```python
from build123d import *

# Parameters (mm, degrees)
SKETCH1_R           = 6
BOSS_EXTRUDE1_DEPTH = 2
SKETCH2_R           = 6
SKETCH2_R_2         = 5.5
BOSS_EXTRUDE2_DEPTH = 2
SKETCH7_W           = 24
SKETCH7_H           = 12
SKETCH7_W_2         = 20
SKETCH7_H_2         = 10
CUT_EXTRUDE1_DEPTH  = 6
SKETCH4_W           = 2.2
SKETCH4_H           = 2.2
CUT_EXTRUDE2_DEPTH  = 2


with BuildPart() as part:
    # Sketch1 → Boss-Extrude1 (new body)
    with BuildSketch(Plane.XY):
        Circle(SKETCH1_R)
    extrude(amount=BOSS_EXTRUDE1_DEPTH)

    # Sketch2 → Boss-Extrude2 (add)
    with BuildSketch(Plane.XY.offset(2)):
        Circle(SKETCH2_R)
        Circle(SKETCH2_R_2, mode=Mode.SUBTRACT)
    extrude(amount=BOSS_EXTRUDE2_DEPTH)

    # Sketch7 → Cut-Extrude1 (cut)
    with BuildSketch(Plane.XY):
        Rectangle(SKETCH7_W, SKETCH7_H)
        Rectangle(SKETCH7_W_2, SKETCH7_H_2, mode=Mode.SUBTRACT)
    extrude(amount=CUT_EXTRUDE1_DEPTH, mode=Mode.SUBTRACT)

    # Sketch4 → Cut-Extrude2 (cut)
    with BuildSketch(Plane.XY):
        Rectangle(SKETCH4_W, SKETCH4_H)
    extrude(amount=CUT_EXTRUDE2_DEPTH, mode=Mode.SUBTRACT)


solid = part.part
```
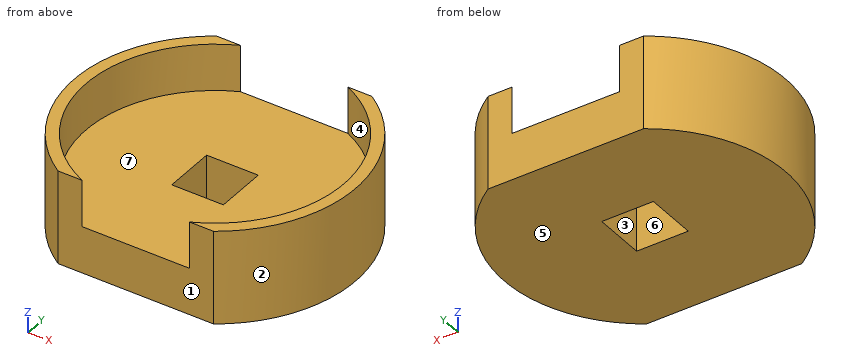
Geometry: final body of the model. Coordinates: model frame, mm. Face numbers are marked on the shaded views. A direction names the side the tool comes from. Round coordinates to 2 decimals unless told otherwise and drop trailing zeros. Write each loop counter-clockwise with the first axis right and the second up, starting at its lowest first coordinate (ties: lowest second). Pieces come first, ordered by that corner, then holes.
Item 1: Material intervals for L1, parallel to Z at x = 1.75, y = -4; L2, parallel to Y at x = 5, z = 1.8; L3, parallel to X at y = 0, z = 2.55, sorted ascending.
Item 2: Section query D-D (x = -3.75). Return loops of the section in (y, z), plus the area to 3 significant figures.
Item 3: Section query B-B (y = 0). Return loops of the section in (x, z), plus the area to 3 significant figures.
Item 4: Pin query (flat end, axial travel): P1, Ø1, axis at x = -2, y = -1, coming from the +Z side. Return the tip coordinate at first contact, or that it passes through.
Item 5: Mould query, pull axis X, two halves, no side actions, for the marked faces 1, 2, 3 and 4. Classes: +X half, -X half, draft (parallel to the pull), parting line (faces both ways), or undercut.
Item 6: Section query A-A (z = 3.25). Return loops of the section in (x, y).
Item 7: Set-up query: the marked faces 5, 6 and 7. Return all of +Z, -Z, +X, -X, +Y, -Y with unobstructed straight access to the full face (end or side cutting, diameter ignored); none if empty.
Item 8: Section query C-C (z = 1.55). Return loops of the section in (x, y), plus the area to 3 significant figures.
Completed:
1. L1: z = 0 to 2
1. L2: y = -3.32 to 3.32
1. L3: x = -6 to -5.5, 5.5 to 6
2. outline: (-4.68, 0) - (4.68, 0) - (4.68, 4) - (4.02, 4) - (4.02, 2) - (-4.02, 2) - (-4.02, 4) - (-4.68, 4) - close
2. area: 21.4 mm2
3. outline: (-6, 0) - (-1.1, 0) - (-1.1, 2) - (-5.5, 2) - (-5.5, 4) - (-6, 4) - close; (1.1, 0) - (6, 0) - (6, 4) - (5.5, 4) - (5.5, 2) - (1.1, 2) - close
3. area: 21.6 mm2
4. P1: stops at z = 2
5. face 1: draft
5. face 2: +X half
5. face 3: undercut
5. face 4: undercut
6. outline: (-3.32, -5) - (-2.29, -5) arc R5.5 cw to (-2.29, 5) - (-3.32, 5) arc R6 ccw to start; (2.29, -5) - (3.32, -5) arc R6 ccw to (3.32, 5) - (2.29, 5) arc R5.5 cw to start
7. face 5: -Z, +X, -X, +Y, -Y
7. face 6: +Z, -Z
7. face 7: +Z
8. outline: (-3.32, -5) - (3.32, -5) arc R6 ccw to (3.32, 5) - (-3.32, 5) arc R6 ccw to start; hole (-1.1, -1.1) - (1.1, -1.1) - (1.1, 1.1) - (-1.1, 1.1) - close
8. area: 99.3 mm2
